Read the model definition and answer for the solid it produces. Units are mm, in the model's axes. Round coordinates to 2 decimals unless told otherwise and drop trailing zeros. Write each loop counter-clockwise with the first axis right and the second up, starting at its lowest first coordinate (ties: lowest second). Pieces come first, ordered by that corner, then holes.
from build123d import *

# Parameters (mm, degrees)
SKETCH_1_W          = 198
SKETCH_1_H          = 50
EXTRUDE_1_DEPTH     = 3
SKETCH_4_W          = 10
SKETCH_4_H          = 5
SKETCH_4_R          = 1.65
EXTRUDE_2_DEPTH     = 5
SKETCH_5_W          = 10
SKETCH_5_H          = 5
SKETCH_5_R          = 1.65
EXTRUDE_3_DEPTH     = 5
SKETCH_6_R          = 1.4
CUT_EXTRUDE_3_DEPTH = 3


with BuildPart() as part:
    # 草图1 → 凸台-拉伸1 (new body)
    with BuildSketch(Plane.XY):
        Rectangle(SKETCH_1_W, SKETCH_1_H)
    extrude(amount=EXTRUDE_1_DEPTH)

    # 草图4 → 凸台-拉伸2 (add)
    with BuildSketch(Plane.ZY.offset(99)):
        with Locations((5, 15)):
            Rectangle(SKETCH_4_W, SKETCH_4_H)
        with Locations((7, 15)):
            Circle(SKETCH_4_R, mode=Mode.SUBTRACT)
        with Locations((5, -15)):
            Rectangle(SKETCH_4_W, SKETCH_4_H)
        with Locations((7, -15)):
            Circle(SKETCH_4_R, mode=Mode.SUBTRACT)
    extrude(amount=-EXTRUDE_2_DEPTH)

    # 草图5 → 凸台-拉伸3 (add)
    with BuildSketch(Plane(origin=(99, 0, 0), x_dir=(0, 0, -1), z_dir=(1, 0, 0))):
        with Locations((-5, 15)):
            Rectangle(SKETCH_5_W, SKETCH_5_H)
        with Locations((-7, 15)):
            Circle(SKETCH_5_R, mode=Mode.SUBTRACT)
        with Locations((-5, -15)):
            Rectangle(SKETCH_5_W, SKETCH_5_H)
        with Locations((-7, -15)):
            Circle(SKETCH_5_R, mode=Mode.SUBTRACT)
    extrude(amount=-EXTRUDE_3_DEPTH)

    # 草图6 → 切除-拉伸3 (cut)
    with BuildSketch(Plane.XY.offset(3)):
        with Locations((-18, 18)):
            Circle(SKETCH_6_R)
        with Locations((18, 18)):
            Circle(SKETCH_6_R)
        with Locations((18, -18)):
            Circle(SKETCH_6_R)
        with Locations((-18, -18)):
            Circle(SKETCH_6_R)
    extrude(amount=-CUT_EXTRUDE_3_DEPTH, mode=Mode.SUBTRACT)


solid = part.part
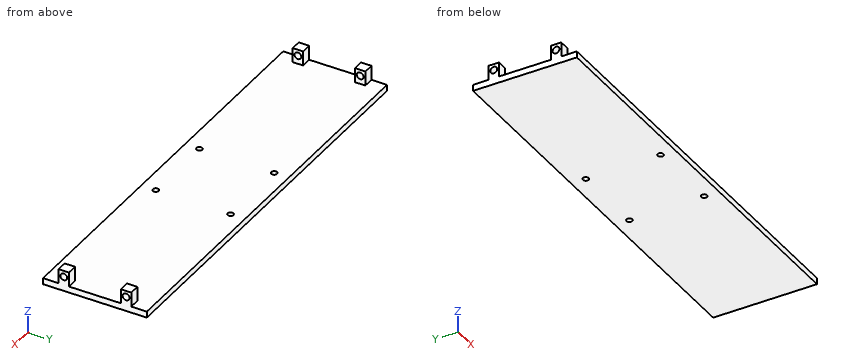
Q1. Section C-C (x = -67) is taken. Determine the outline of the cut face in (y, z), then the cut area to 3 significant figures.
Verdict:
outline: (-25, 0) - (25, 0) - (25, 3) - (-25, 3) - close
area: 150 mm2
Q2. Flat-ended cylindrical pins translate along their axes: pin 1 Ø6 at (x, y) = (0, 2.5) entering from +Z; pin 2 Ø5.5 at (x, z) = (97, 7.5) entering from -Y; pin 3 Ø2.5 at (x, z) = (97.5, 8) entering from +Y. Find the tip coordinate at first contact, or state that the pin passes through.
Verdict:
pin 1: stops at z = 3
pin 2: stops at y = -17.5
pin 3: stops at y = 17.5
Q3. Section A-A (z = 7) is taken. State how many separate pieces and enclosed holes the cut face has, then the cut area to 3 significant figures.
Verdict:
separate pieces: 8
enclosed holes: 0
area: 34.0 mm2
Q4. Straight lines are drawn through the part: probe 1 along Y at (x, z) = (-18, 1.25); probe 2 along Y at (x, z) = (96, 7); probe 3 along X at (y, z) = (15.5, 4.5). For each, find the intervals that lie inside material, in ascending order.
Verdict:
probe 1: y = -25 to -19.4, -16.6 to 16.6, 19.4 to 25
probe 2: y = -17.5 to -16.65, -13.35 to -12.5, 12.5 to 13.35, 16.65 to 17.5
probe 3: x = -99 to -94, 94 to 99
Q5. Section B-B (y = -5) is taken. Determine the outline of the cut face in (x, z), then the cut area to 3 significant figures.
Verdict:
outline: (-99, 0) - (99, 0) - (99, 3) - (-99, 3) - close
area: 594 mm2
